For this review, take the finished solid that the model builds, in its own axes (mm). Give positions to 0.01 mm unless a question says otherwise; leave off trailing zeros. Write each loop counter-clockwise with the first axis right and the second up, starting at its lowest first coordinate (ties: lowest second). Pieces come first, ordered by that corner, then holes. Notation, with made-up numbers: M -39.75,-10 L -13.75,-10 A22 ccw -13.75,21 Z; hole C -12.75,-0.5 d8. An arc over 180 degrees is marked long. One line per item, written item: value. Start each with the question number.
Item 1: Consider section B-B, the plane z = -27.5. Write out the cut boundary in (x, y), and give its area (3 significant figures).
Item 2: To check wall thickness, follow probe 1 along X at (y, z) = (6.75, 0); probe 2 along Z at (x, y) = (23, 2.5); probe 3 along X at (y, z) = (9.5, -75). State the ranges of each line that lie inside material, in increasing order.
Item 3: Consider section D-D, the plane x = 65.5. Write out the cut boundary in (y, z).
Item 4: Consider section C-C, the plane z = 35. Write out the cut boundary in (x, y), and give its area (3 significant figures).
Item 5: Consider section A-A, the plane y = 3.5. Write out the cut boundary in (x, z), and give its area (3 significant figures).
Item 6: Clearance check with flat-ended pins moving along their axes: pin 1 Ø1 at (y, z) = (6, -27) entering from -X; pin 2 Ø1.5 at (y, z) = (4, -43) entering from -X; pin 3 Ø2 at (x, y) = (15, 3) entering from +Z. State where each tip first meets the part, or that it passes through.
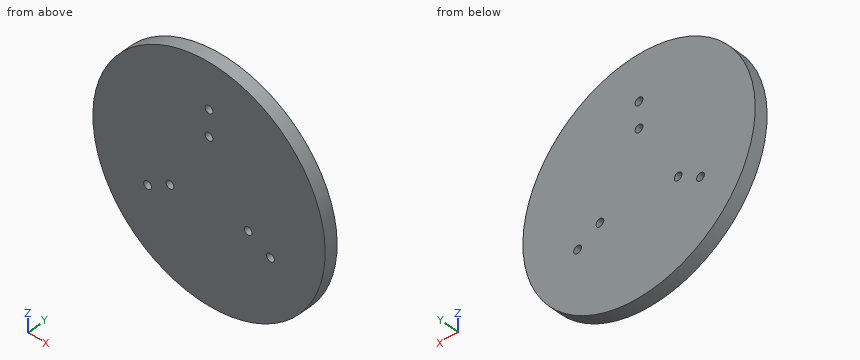
```python
from build123d import *

# Parameters (mm, degrees)
F0_W     = 180
F0_H     = 180
F1_DEPTH = 10
F2_R     = 3
F3_DEPTH = 10.001
F5_DEPTH = 10.001


with BuildPart() as f1:
    # F0 (on Front) → F1 (new body)
    with BuildSketch(Plane.XZ):
        Rectangle(F0_W, F0_H)
    extrude(amount=-F1_DEPTH)

    # F2 (on face) → F3 (cut, through all)
    with BuildSketch(Plane.XZ):
        with Locations((0, 55)):
            Circle(F2_R)
        with Locations((0, 35)):
            Circle(F2_R)
        with Locations((-30.3108891325, -17.5)):
            Circle(F2_R)
        with Locations((-47.6313972081, -27.5)):
            Circle(F2_R)
        with Locations((30.3108891325, -17.5)):
            Circle(F2_R)
        with Locations((47.6313972081, -27.5)):
            Circle(F2_R)
    extrude(amount=-F3_DEPTH, mode=Mode.SUBTRACT)

    # F4 (on face) → F5 (cut, through all)
    with BuildSketch(Plane.XZ):
        with BuildLine():
            ThreePointArc((-90, 2.079e-07), (-63.6396103357, 63.6396102779), (-2.896e-07, 90))
            Line((-2.896e-07, 90), (-90, 90))
            Line((-90, 90), (-90, 2.079e-07))
        make_face()
        with BuildLine():
            ThreePointArc((-2.896e-07, 90), (63.6396102044, 63.6396104092), (90, 0))
            Line((90, 0), (90, 90))
            Line((90, 90), (-2.896e-07, 90))
        make_face()
        with BuildLine():
            Line((90, -90), (90, 0))
            ThreePointArc((90, 0), (63.6396104617, -63.6396101519), (4.381e-07, -90))
            Line((4.381e-07, -90), (90, -90))
        make_face()
        with BuildLine():
            Line((-90, -90), (4.381e-07, -90))
            ThreePointArc((4.381e-07, -90), (-63.6396102254, -63.6396103882), (-90, 2.079e-07))
            Line((-90, 2.079e-07), (-90, -90))
        make_face()
    extrude(amount=-F5_DEPTH, mode=Mode.SUBTRACT)


solid = f1.part
```
Model answer:
1. outline: M -85.7,0 L -50.63,0 L -50.63,10 L -85.7,10 Z; M -44.63,0 L 44.63,0 L 44.63,10 L -44.63,10 Z; M 50.63,0 L 85.7,0 L 85.7,10 L 50.63,10 Z
1. area: 1,590 mm2
2. probe 1: x = -90 to 90
2. probe 2: z = -87.01 to 87.01
2. probe 3: x = -49.75 to 49.75
3. outline: M 0,-61.72 L 10,-61.72 L 10,61.72 L 0,61.72 Z
4. outline: M -82.92,0 L -3,0 L -3,10 L -82.92,10 Z; M 3,0 L 82.92,0 L 82.92,10 L 3,10 Z
4. area: 1,600 mm2
5. outline: C 0,0 d180; hole C -47.63,-27.5 d6; hole C -30.31,-17.5 d6; hole C 0,35 d6; hole C 0,55 d6; hole C 30.31,-17.5 d6; hole C 47.63,-27.5 d6
5. area: 25,300 mm2
6. pin 1: stops at x = -86.01
6. pin 2: stops at x = -79.47
6. pin 3: stops at z = 88.9
